Solid Edge part; units mm, degrees
sketch "Sketch1" plane through (0, 0, 0) normal (0, 0, 1) x (1, 0, 0)
  line L0 (-27.5, -27.5) -> (27.5, -27.5)
  line L1 (27.5, -27.5) -> (27.5, 27.5)
  line L2 (27.5, 27.5) -> (-27.5, 27.5)
  line L3 (-27.5, 27.5) -> (-27.5, -27.5)
extrude "Protrusion1" add sketch "Sketch1" along normal up to vertex (38.8909 mm away)
sketch "Sketch2" plane through (0, 0, 0) normal (1, 0, 0) x (0, 1, 0)
  line L0 (-27.5, 0) -> (0, 38.8909)
extrude "Cutout1" cut sketch "Sketch2" along normal mid plane 82.5125 material side at (0, -13.7908, 19.4743)
pattern_circular "Pattern1" count 4 over 360 about axis through (0, 0, 0) along (0, 0, -1) of "Cutout1"
The listing builds one solid part. Answer for the finished solid, in the listing's coordinates (mm). Coordinates: 2 decimals unless noted, no trailing zeros. Loops run counter-clockwise (first coordinate to the right, second up) from the corner with the lowest first, then second, coordinate; pieces in that order, holes last. Notation, with made-up numbers: (20, 0.25) - (38, 0.25) arc R20 cw to (38, 37.25) - close; hole circle Ø5 at (-11, 6). An arc over 180 degrees is marked (long way). Write item = value, one per line.
1) Find the intervals of material crossed by line 1 along Y through (x, z) = (3.5, 9); line 2 along Z through (x, y) = (-1, 20.5); line 3 along Z through (x, y) = (21, -16.5), in increasing order.
Responses:
line_1 = -21.14 to 21.14
line_2 = 0 to 9.9
line_3 = 0 to 9.19
2) Section B-B (y = -22.5) is taken. Determine the outline of the cut face in (x, z).
Responses:
outline = (-27.5, 0) - (27.5, 0) - (22.5, 7.07) - (-22.5, 7.07) - close
3) Section A-A (z = 24) is taken. Determine the outline of the cut face in (x, y), plus the area to 3 significant figures.
Responses:
outline = (-10.53, -10.53) - (10.53, -10.53) - (10.53, 10.53) - (-10.53, 10.53) - close
area = 443 mm^2
4) Each of these flat-tipped pins is pushed along its axis until it touches: P1, Ø8, axis at x = -18.5, y = 1.5, coming from the +Z side; P2, Ø3, axis at y = 3, z = 7.5, coming from the -X side; P3, Ø10, axis at x = -9.5, z = 30.5, coming from the +Y side. Where does it stop, or does it pass through?
Responses:
P1 = 18.38
P2 = -23.26
P3 = 9.47
